Source: CAD feature listing. Evaluate the final solid. Frame: model axes, mm. Face numbers are marked on the shaded views. A direction names the side the tool comes from. Round coordinates to 2 decimals unless told otherwise and drop trailing zeros. Order: outer loops, then holes, each group sorted by start corner. A loop starts at its lowest first (then second) coordinate and runs counter-clockwise, first axis right, second up. Notation, with made-up numbers: (35, 53) -> (61, 53) arc R10 cw to (61, 68) -> close; hole circle Ø5 at (68.25, 60). An arc over 180 degrees is marked (long way). Answer as CSV lines item,"result". Start each with the question number.
(1) Section query A-A (z = -15). Count the separate pieces of the cut face and the enclosed holes in it, plus the area to 3 significant figures.
(2) Section query C-C (x = 25). Output: boundary loops of the cut face in (y, z) (3 decimals), plus the area to 3 significant figures.
(3) Set-up query: the marked faces 5, 6, 7, 8 and 9. Return all of +Z, -Z, +X, -X, +Y, -Y with unobstructed straight access to the full face (end or side cutting, diameter ignored); none if empty.
(4) Pull-direction query (Z, two-part tool) for the marked faces 1, 2, 3 and 4; classes: +Z half, -Z half, draft (parallel to the pull), parting line (faces both ways), or undercut.
(5) Line query: line 1 along Z through (x, y) = (22.5, 15.06) (3 decimals); line 2 along Z through (x, y) = (10.5, 3); line 3 along Y through (x, z) = (24, -15) (3 decimals). Output: solid intervals per line, ascending. Write a range as from..to.
(6) Contact query for flat-ended pins moving along their axis: P1, Ø4, axis at x = 2.5, z = 23.5, coming from the -Y side; P2, Ø10, axis at y = 113, z = 10, coming from the -X side (3 decimals); P3, Ø7.5, axis at y = 8, z = -16.5, coming from the -X side; P4, Ø3, axis at y = 23.56, z = -15, coming from the +X side. Output: stop coordinate, or through.
(7) Section query B-B (y = 6.56). Output: boundary loops of the cut face in (x, z).
(8) Section query D-D (x = 18). Output: boundary loops of the cut face in (y, z), plus the area to 3 significant figures.
Autodesk Inventor part; units mm, degrees
ref_plane "Work Plane1" through (0, 0, -15) normal (0, 0, 1) x (1, 0, 0)
ref_plane "YZ Plane" through (0, 0, 0) normal (1, 0, 0) x (0, 1, 0)
ref_plane "XZ Plane" through (0, 0, 0) normal (0, 1, 0) x (-1, 0, 0)
sketch "Sketch1" plane through (0, 0, 0) normal (0, 0, 1) x (1, 0, 0)
  line L0 (0, 0) -> (25, 0)
  line L1 (25, 0) -> (25, 40)
  line L2 (25, 40) -> (0, 40)
  line L3 (0, 40) -> (0, 0)
  dimension "d1" = 25
  dimension "d2" = 40
  dimension "d3" = 25
extrude "Extrusion1" add sketch "Sketch1" against normal blind 30
sketch "Sketch2" plane through (25, 0, 0) normal (1, 0, 0) x (0, 0, -1)
  line L0 (0, 0) -> (30, 0)
  circle A0 centre (15, 6.56) radius 2.46
extrude "Extrusion2" cut sketch "Sketch2" against normal blind 30
sketch "Sketch3" plane through (0, 0, 0) normal (-1, 0, 0) x (0, 0, 1)
  line L0 (0, 0) -> (-30, 0)
  line L1 (-25.05, 0) -> (-4.95, 0)
  line L2 (-4.95, 0) -> (-4.95, 33.12)
  line L3 (-4.95, 33.12) -> (-25.05, 33.12)
  line L4 (-25.05, 33.12) -> (-25.05, 0)
  dimension "d11" = 20.1
extrude "Extrusion3" cut sketch "Sketch3" against normal blind 20
sketch "Sketch4" plane through (0, 0, 0) normal (0, -1, 0) x (1, 0, 0)
  line L0 (20, -4.95) -> (20, -25.05)
  line L1 (20, -15) -> (25, -15)
  line L2 (25, 0) -> (25, -30)
  line L3 (20, -8.025) -> (25, -8.025)
  line L4 (25, -8.025) -> (25, -21.975)
  line L5 (25, -21.975) -> (20, -21.975)
  line L6 (20, -21.975) -> (20, -8.025)
  line L7 (20, -8.025) -> (25, -21.975) construction
  line L8 (25, -8.025) -> (20, -21.975) construction
  line L9 (25, -12.54) -> (25, -17.46)
  point P0 (0, 0)
  point P1 (22.5, -15)
  dimension "d14" = 13.95
extrude "Extrusion4" add sketch "Sketch4" along normal blind 15
sketch "Sketch5" plane through (20, 0, 0) normal (-1, 0, 0) x (0, 0, 1)
  circle A0 centre (-15, 6.56) radius 2.46
  circle A1 centre (-15, 6.56) radius 4.7025
  circle A2 centre (-15, 6.56) radius 2.46
  circle A3 centre (-15, 6.56) radius 2.46
  point P0 (0, 0)
  dimension "d17" = 9.405
extrude "Extrusion5" cut sketch "Sketch5" against normal blind 2.1
sketch "Sketch6" plane through (25, 0, 0) normal (1, 0, 0) x (0, 0, -1)
  circle A0 centre (15, 6.56) radius 4.7025
  line L0 (15, 6.56) -> (15, 23.56)
  circle A1 centre (15, 23.56) radius 2.46
  point P0 (0, 0)
  dimension "d20" = 17
  dimension "d21" = 4.92
extrude "Extrusion6" cut sketch "Sketch6" against normal blind 10 contours A1
sketch "Sketch7" plane through (20, 0, 0) normal (-1, 0, 0) x (0, 0, 1)
  circle A0 centre (-15, 23.56) radius 2.46
  circle A1 centre (-15, 23.56) radius 4.7025
  point P0 (0, 0)
  dimension "d24" = 9.405
extrude "Extrusion7" cut sketch "Sketch7" against normal blind 2.1
sketch "Sketch9" plane through (25, 0, 0) normal (1, 0, 0) x (0, 0, -1)
  circle A0 centre (15, 6.56) radius 2.46
  circle A1 centre (15, 6.56) radius 2.46
  circle A2 centre (15, 23.56) radius 2.46
  circle A3 centre (15, 23.56) radius 2.46
  line L0 (30, 40) -> (30, 0)
  line L1 (30, 0) -> (30, 40)
  line L2 (30, 40) -> (0, 40)
  line L3 (0, 40) -> (0, 0)
  line L4 (0, 0) -> (8.025, 0)
  line L5 (21.975, 0) -> (21.975, -15)
  line L6 (21.975, -15) -> (8.025, -15)
  line L7 (8.025, -15) -> (8.025, 0)
  line L8 (0, 0) -> (8.025, 0)
  line L9 (21.975, 0) -> (30, 0)
extrude "Extrusion8" add sketch "Sketch9" along normal blind 5
sketch "Sketch10" plane through (0, 40, 0) normal (0, 1, 0) x (1, 0, 0)
  line L0 (0, 30) -> (30, 30)
  line L1 (30, 0) -> (0, 0)
  line L2 (0, 30) -> (30, 30)
  line L3 (30, 30) -> (30, 0)
  line L4 (30, 0) -> (0, 0)
  line L5 (0, 0) -> (0, 30)
extrude "Extrusion9" add sketch "Sketch10" along normal blind 30
sketch "Sketch12" plane through (30, 0, 0) normal (1, 0, 0) x (0, 0, -1)
  circle A0 centre (15, 6.56) radius 2.46
  line L0 (15, 6.56) -> (15, 15.06)
  circle A1 centre (15, 15.06) radius 2.525
  point P0 (0, 0)
  dimension "d31" = 8.5
  dimension "d33" = 5.05
extrude "Extrusion10" cut sketch "Sketch12" against normal blind 30 contours A1
sketch "Sketch14" plane through (0, 0, 0) normal (0, 0, 1) x (1, 0, 0)
  line L0 (30, 70) -> (0, 70)
  line L1 (0, 70) -> (0, 85)
  line L2 (30, 0) -> (30, 70)
  line L3 (30, 118) -> (30, 70)
  line L4 (30, 105) -> (30, 100)
  line L5 (-7, 134) -> (-12, 136)
  line L6 (-7, 102) -> (-12, 100)
  line L7 (-7, 102) -> (-2, 118)
  line L8 (-2, 118) -> (-7, 134)
  line L9 (15, 136) -> (30, 118)
  line L10 (-12, 136) -> (15, 136)
  line L11 (0, 85) -> (0, 100)
  line L12 (0, 100) -> (-12, 100)
  point P0 (0, 0)
  dimension "d82" = 12
extrude "Extrusion12" add sketch "Sketch14" against normal blind 30
sketch "Sketch15" plane through (0, 0, -25.05) normal (-1, 0, 0) x (0, 0, 1)
  line L0 (0, 33.12) -> (20.1, 33.12)
  line L1 (20.1, 33.12) -> (20.1, 0)
  line L2 (0, 33.12) -> (20.1, 33.12)
  line L3 (20.1, 33.12) -> (20.1, 31.1)
  line L4 (20.1, 31.1) -> (0, 31.1)
  line L5 (0, 31.1) -> (0, 33.12)
  point P0 (25.05, 0)
  dimension "d57" = 2.02
extrude "Extrusion13" add sketch "Sketch15" against normal blind 20
sketch "Sketch23" plane through (0, 0, 0) normal (0, 0, 1) x (1, 0, 0)
  line L0 (0, 100) -> (-12, 100)
  line L1 (0, 100) -> (-12, 100)
  line L2 (-12, 100) -> (-7, 102)
  line L3 (-12, 100) -> (-7, 102)
  line L4 (-7, 102) -> (-2, 118)
  line L5 (-7, 102) -> (-2, 118)
  line L6 (-2, 118) -> (-7, 134)
  line L7 (-2, 118) -> (-7, 134)
  line L8 (-12, 136) -> (15, 136)
  line L9 (-7, 134) -> (-12, 136)
  line L10 (-12, 136) -> (15, 136)
  line L11 (15, 136) -> (30, 118)
  line L12 (15, 136) -> (30, 118)
  line L13 (30, 118) -> (30, 88)
  line L14 (30, 0) -> (30, 118)
  line L15 (30, 88) -> (0, 88)
  line L16 (0, 88) -> (0, 100)
  point P0 (0, 0)
  dimension "d83" = 30
  dimension "d84" = 30
extrude "Extrusion14" add sketch "Sketch23" along normal blind 45
ref_plane "Work Plane1" through (0, 0, -15) normal (0, 0, 1) x (1, 0, 0)
mirror "Mirror1" about plane through (0, 0, -15) normal (0, 0, 1) of "Extrusion14"
properties part number "rec_b_32mm_x_120mm"
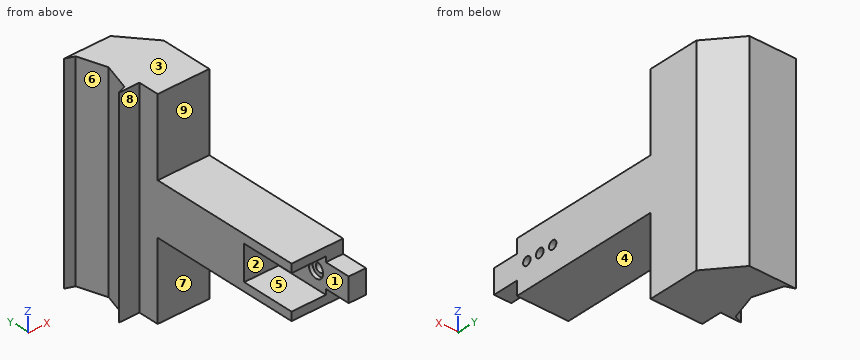
Answer block:
1,separate pieces,"4"
1,enclosed holes,"0"
1,area,"3,490 mm2"
2,outline,"(-15, -21.975) -> (0, -21.975) -> (0, -30) -> (88, -30) -> (88, -75) -> (124, -75) -> (124, 45) -> (88, 45) -> (88, 0) -> (0, 0) -> (0, -8.025) -> (-15, -8.025) -> close; hole circle Ø4.92 at (6.56, -15); hole circle Ø5.05 at (15.06, -15); hole circle Ø4.92 at (23.56, -15)"
2,area,"7,110 mm2"
3,face 5,"-X, -Y"
3,face 6,"+Z, -Z, -X"
3,face 7,"-Z, +X, -X, -Y"
3,face 8,"+Z, -Z, -X, -Y"
3,face 9,"+Z, +X, -X, -Y"
4,face 1,"undercut"
4,face 2,"undercut"
4,face 3,"+Z half"
4,face 4,"-Z half"
5,line 1,"-30..-17.525, -12.475..0"
5,line 2,"-30..-25.05, -4.95..0"
5,line 3,"-15..4.1, 9.02..12.535, 17.585..21.1, 26.02..125.2"
6,P1,"y = 88"
6,P2,"x = -5.125"
6,P3,"x = 20"
6,P4,"through"
7,outline,"(0, -30) -> (30, -30) -> (30, -17.46) -> (22.1, -17.46) -> (22.1, -19.7) -> (20, -19.7) -> (20, -25.05) -> (0, -25.05) -> close; (0, -4.95) -> (20, -4.95) -> (20, -10.3) -> (22.1, -10.3) -> (22.1, -12.54) -> (30, -12.54) -> (30, 0) -> (0, 0) -> close"
8,outline,"(0, -30) -> (88, -30) -> (88, -75) -> (132.4, -75) -> (132.4, 45) -> (88, 45) -> (88, 0) -> (0, 0) -> (0, -4.95) -> (31.1, -4.95) -> (31.1, -25.05) -> (0, -25.05) -> close"
8,area,"7,340 mm2"
